```python
from build123d import *

# Parameters (mm, degrees)
F0_R         = 5
F1_DEPTH     = 75
F2_R         = 7
F2_R_2       = 5
F4_DEPTH     = 25
F3_R         = 7
F3_R_2       = 5
F5_DEPTH     = 25
F6_S5_R      = 5
F6_T6_DEPTH  = 12
F6_S11_R     = 5
F6_T12_DEPTH = 12
F7_R         = 5.05
F8_DEPTH     = 11
F9_R         = 5.05
F10_DEPTH    = 11


# Not quite as in the source:
# - a fillet or chamfer that OpenCascade refuses, or shapes differently, is made with other operations: its cross-section is extruded or revolved along the edge and cut away or added


with BuildPart() as f1:
    # F0 (on Top) → F1 (new body, symmetric)
    with BuildSketch(Plane.XY):
        Circle(F0_R)
    extrude(amount=F1_DEPTH, both=True)

    # F2 (on face) → F4 (join)
    with BuildSketch(Plane.XY.offset(75)):
        Circle(F2_R)
        Circle(F2_R_2, mode=Mode.SUBTRACT)
        Circle(F2_R_2)
    extrude(amount=F4_DEPTH)

    # F3 (on face) → F5 (join)
    with BuildSketch(Plane(origin=(0, 0, -75), x_dir=(1, 0, 0), z_dir=(0, 0, -1))):
        Circle(F3_R)
        Circle(F3_R_2, mode=Mode.SUBTRACT)
        Circle(F3_R_2)
    extrude(amount=F5_DEPTH)

    # F6: chamfer of 8 x 2.1435935394 on 2 edges, made by hand


with BuildPart() as f6_tool2:
    # F6_s3 → F6_t4 (revolve)
    with BuildSketch(Plane.XZ):
        Polygon((7, -83), (4.8564064606, -75), (7, -75), align=None)
    revolve(axis=Axis((0, 0, -75), (0, 0, -1)))

    # F6_s5 → F6_t6 (cut, symmetric)
    with BuildSketch(Plane.XY.offset(-79)):
        Circle(F6_S5_R)
    extrude(amount=F6_T6_DEPTH, both=True, mode=Mode.SUBTRACT)


with BuildPart() as f1_1:
    add(f1.part)

    # F6_t1: cut F6_tool2
    add(f6_tool2.part, mode=Mode.SUBTRACT)


with BuildPart() as f6_tool8:
    # F6_s9 → F6_t10 (revolve)
    with BuildSketch(Plane.XZ):
        Polygon((4.8564064606, 75), (7, 83), (7, 75), align=None)
    revolve(axis=Axis((0, 0, 75), (0, 0, 1)))

    # F6_s11 → F6_t12 (cut, symmetric)
    with BuildSketch(Plane.XY.offset(79)):
        Circle(F6_S11_R)
    extrude(amount=F6_T12_DEPTH, both=True, mode=Mode.SUBTRACT)


with BuildPart() as f1_2:
    add(f1_1.part)

    # F6_t7: cut F6_tool8
    add(f6_tool8.part, mode=Mode.SUBTRACT)

    # F7 (on face) → F8 (cut)
    with BuildSketch(Plane(origin=(0, 0, -100), x_dir=(1, 0, 0), z_dir=(0, 0, -1))):
        Circle(F7_R)
    extrude(amount=-F8_DEPTH, mode=Mode.SUBTRACT)

    # F9 (on face) → F10 (cut)
    with BuildSketch(Plane.XY.offset(100)):
        Circle(F9_R)
    extrude(amount=-F10_DEPTH, mode=Mode.SUBTRACT)


solid = f1_2.part
```
The listing builds one solid part. Answer for the finished solid, in the listing's coordinates (mm). A direction names the side the tool comes from. Give positions to 0.01 mm unless a question says otherwise; leave off trailing zeros. Write each loop counter-clockwise with the first axis right and the second up, starting at its lowest first coordinate (ties: lowest second). Pieces come first, ordered by that corner, then holes. Notation, with made-up numbers: (-7.5, 55) -> (29.5, 55) arc R35 ccw to (29.5, 94) -> close; hole circle Ø8 at (-7.5, 80.5). An arc over 180 degrees is marked (long way). Write item = value, one per line. Start each with the question number.
1) Which of the six approach directions +Z, -Z, +X, -X, +Y, -Y give full straight-line access (tool end or side, diameter ignored) to faces 1 (the face through (4.817, -1.517, -94.577)), 2 (the face through (5.312, 1.673, 77.662)), 3 (the face through (0, 0, 89)), 4 (the face through (6.466, -2.681, 91.381))?
2) Determine the mould class of faces 5 (the face through (-0.721, -5.494, -77.557)), 6 (the face through (3, 4, 1)), 7 (the face through (2, 5, -100)), 8 (the face through (4.817, 1.517, 94.577)) for opening direction Z: +Z half, -Z half, draft (parallel to the pull), parting line (faces both ways), or undercut.
3) Straight lines are drawn through the part: line 1 along Y through (x, z) = (0, -96.75); line 2 along Z through (x, y) = (-4.5, 2). For each, find the intervals that lie inside material, in ascending order.
4) The part is cut by section A-A, the plane y = 0. Determine the outline of the cut face in (x, z).
5) Each of these flat-tipped pins is pushed along its axis until it touches: pin 1 (6 mm diameter, centred on x = 0, y = 0, fed in from +Z); pin 2 (5 mm diameter, centred on x = 2.5, z = -32.5, fed in from +Y); pin 3 (8 mm diameter, centred on x = 0, y = 0, fed in from -Z). Where does it stop, or does it pass through?
6) The part is cut by section C-C, the plane z = -26.5. Determine the outline of the cut face in (x, y), and give its area (3 significant figures).
Solutions:
q1.face_1 = -Z
q1.face_2 = none
q1.face_3 = +Z
q1.face_4 = +Z, -Z
q2.face_5 = undercut
q2.face_6 = undercut
q2.face_7 = -Z half
q2.face_8 = draft
q3.line_1 = -7 to -5.05, 5.05 to 7
q3.line_2 = -89 to 89
q4.outline = (-7, -100) -> (-5.05, -100) -> (-5.05, -89) -> (5.05, -89) -> (5.05, -100) -> (7, -100) -> (7, -83) -> (5, -75.54) -> (5, 75.54) -> (7, 83) -> (7, 100) -> (5.05, 100) -> (5.05, 89) -> (-5.05, 89) -> (-5.05, 100) -> (-7, 100) -> (-7, 83) -> (-5, 75.54) -> (-5, -75.54) -> (-7, -83) -> close
q5.pin_1 = 89
q5.pin_2 = 5
q5.pin_3 = -89
q6.outline = circle Ø10 at (0, 0)
q6.area = 78.5 mm²
